Source: three-view drawing plus pictorial views. Frame: mm from the lowest corner of the part. A direction names the side the tool comes from. Give positions to 0.01 mm unless a question says otherwise; leave off trailing zeros. Order: outer loops, then holes, each group sorted by start corner. A loop starts at its lowest first (then second) coordinate and runs counter-clockwise, first axis right, second up. Notation, with made-up numbers: (10.25, -12.75) - (62.25, -12.75) arc R14 ccw to (62.25, 10.25) - close; hole circle Ø8 at (-4.5, 15). An arc over 180 degrees is marked (long way). Answer in a Markdown table with one row per item. Add a question column.
1. Section query C-C on y = 23. Return loops of the section in (x, z).
2. Mould query, pull axis X, two halves, no side actions, for the marked faces 1, 2, 3 and 4. Classes: released by +X, released by -X, zero draft, split by the parting line, or undercut.
3. Access query for the marked faces 5, 6, 7 and 8. Directions: +Z, -Z, +X, -X, +Y, -Y. A direction counts if a zero-diameter tool reaches every point of the face in a straight line with its end or side. Return the directions, or none.
4. Section query D-D on y = 120. Return loops of the section in (x, z), and give its area (3 significant figures).
5. Section query B-B on z = 116. Return loops of the section in (x, y), and give its area (3 significant figures).
6. Ray query, line 1 (Z direction, x = 88.5, y = 60); line 2 (Y direction, x = 101.5, z = 115.5); line 3 (Y direction, x = 19.5, z = 80). Return the intervals inside material, ascending. Write a range as [from, to].
7. Section query A-A on x = 100. Return loops of the section in (y, z), and give its area (3 significant figures).
8. Contact query for flat-ended pins moving along their axis: pin 1 (2 mm diameter, centred on x = 94, y = 58, fed in from +Z); pin 2 (5 mm diameter, centred on y = 129.5, z = 49.5, fed in from +X); pin 3 (6 mm diameter, centred on y = 131.5, z = 23.5, fed in from -X); pin 4 (2 mm diameter, centred on x = 73, z = 79, fed in from -Y). Output: stop coordinate, or through.
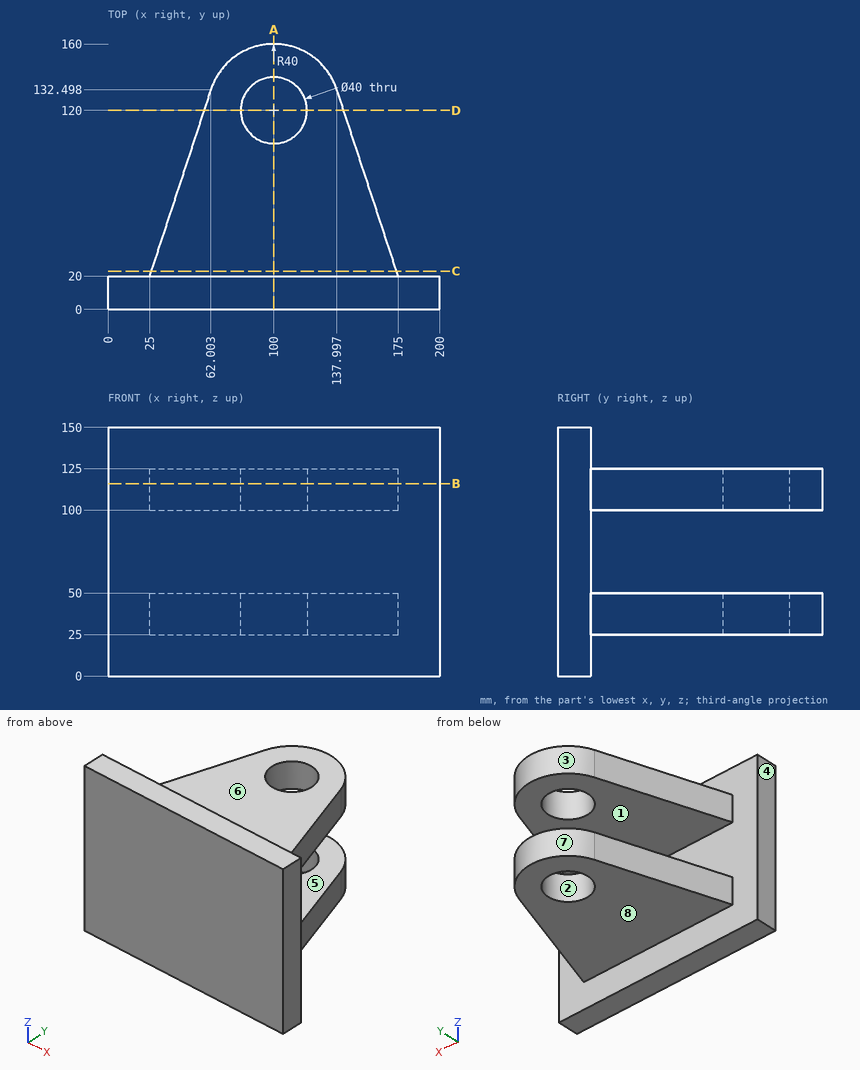
Answer:
| question | item | result |
|---|---|---|
| 1 | outline | (25.99, 25) - (174.01, 25) - (174.01, 50) - (25.99, 50) - close; (25.99, 100) - (174.01, 100) - (174.01, 125) - (25.99, 125) - close |
| 2 | face 1 | zero draft |
| 2 | face 2 | undercut |
| 2 | face 3 | split by the parting line |
| 2 | face 4 | released by -X |
| 3 | face 5 | +X, -X, +Y |
| 3 | face 6 | +Z, +X, -X, +Y |
| 3 | face 7 | +Z, -Z, +Y |
| 3 | face 8 | -Z, +X, -X, +Y |
| 4 | outline | (57.89, 25) - (80, 25) - (80, 50) - (57.89, 50) - close; (57.89, 100) - (80, 100) - (80, 125) - (57.89, 125) - close; (120, 25) - (142.11, 25) - (142.11, 50) - (120, 50) - close; (120, 100) - (142.11, 100) - (142.11, 125) - (120, 125) - close |
| 4 | area | 2,210 mm² |
| 5 | outline | (0, 0) - (200, 0) - (200, 20) - (175, 20) - (138, 132.5) arc R40 ccw to (62, 132.5) - (25, 20) - (0, 20) - close; hole circle Ø40 at (100, 120) |
| 5 | area | 17,000 mm² |
| 6 | line 1 | z = [25, 50], [100, 125] |
| 6 | line 2 | y = [0, 100.06], [139.94, 159.97] |
| 6 | line 3 | y = [0, 20] |
| 7 | outline | (0, 0) - (20, 0) - (20, 25) - (100, 25) - (100, 50) - (20, 50) - (20, 100) - (100, 100) - (100, 125) - (20, 125) - (20, 150) - (0, 150) - close; (140, 25) - (160, 25) - (160, 50) - (140, 50) - close; (140, 100) - (160, 100) - (160, 125) - (140, 125) - close |
| 7 | area | 8,000 mm² |
| 8 | pin 1 | stops at z = 125 |
| 8 | pin 2 | stops at x = 139.81 |
| 8 | pin 3 | stops at x = 60.82 |
| 8 | pin 4 | stops at y = 0 |
